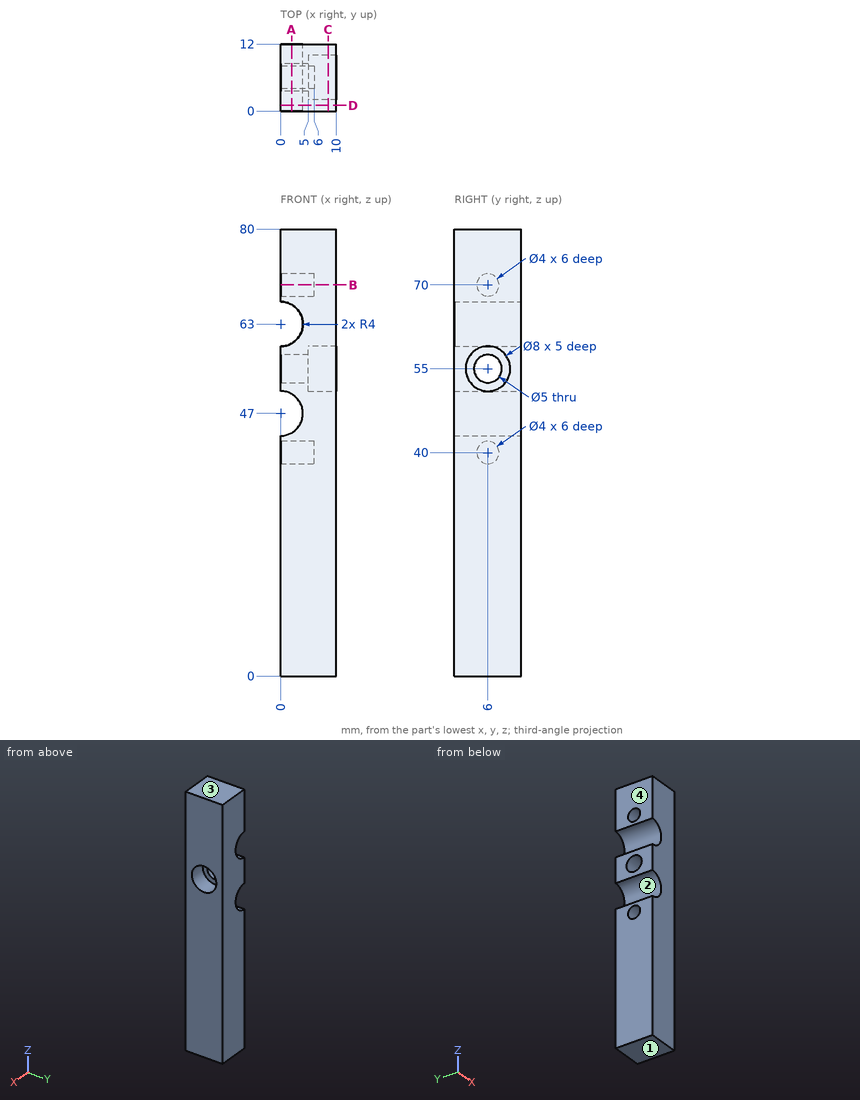
Job drawing, mm, ordinate dimensions from the low corner. One solid piece. Round coordinates to 2 decimals unless told otherwise and drop trailing zeros. Loops run counter-clockwise (first coordinate to the right, second up) from the corner with the lowest first, then second, coordinate; pieces in that order, holes last. Notation, with made-up numbers: (30.25, -18.5) -> (43.25, -18.5) arc R25 cw to (43.25, -0.5) -> close; hole circle Ø1 at (45.25, -34.5). An arc over 180 degrees is marked (long way). Use a Markdown table: item, result.
1) Cut at C-C, the plane x = 8.5. List the corners of the cut face in (y, z).
The answers:
| item | result |
|---|---|
| outline | (0, 0) -> (12, 0) -> (12, 80) -> (0, 80) -> close; hole circle Ø8 at (6, 55) |
2) Drop a flat-ended pin along its axis: pin 1 Ø6 at (y, z) = (6, 55) entering from +X. Give the stop position or say it passes through.
The answers:
| item | result |
|---|---|
| pin 1 | stops at x = 5 |
3) Cut at A-A, the plane x = 2. List the corners of the cut face in (y, z).
The answers:
| item | result |
|---|---|
| outline | (0, 0) -> (12, 0) -> (12, 43.54) -> (0, 43.54) -> close; (0, 50.46) -> (12, 50.46) -> (12, 59.54) -> (0, 59.54) -> close; (0, 66.46) -> (12, 66.46) -> (12, 80) -> (0, 80) -> close; hole circle Ø5 at (6, 55); hole circle Ø4 at (6, 40); hole circle Ø4 at (6, 70) |
4) Cut at B-B, the plane z = 70. List the corners of the cut face in (x, y).
The answers:
| item | result |
|---|---|
| outline | (0, 0) -> (10, 0) -> (10, 12) -> (0, 12) -> (0, 8) -> (6, 8) -> (6, 4) -> (0, 4) -> close |
5) Cut at D-D, the plane y = 1. List the corners of the cut face in (x, z), and give its area (3 significant figures).
The answers:
| item | result |
|---|---|
| outline | (0, 0) -> (10, 0) -> (10, 80) -> (0, 80) -> (0, 67) arc R4 cw to (0, 59) -> (0, 51) arc R4 cw to (0, 43) -> close |
| area | 750 mm2 |
6) Pull direction Z, two halves, no side cores. Call the marked faces 1, 2, 3 and 4: pulls with the +Z half, pulls with the -Z half, needs draft (parallel to the pull), parting line crosses it, or undercut.
The answers:
| item | result |
|---|---|
| face 1 | pulls with the -Z half |
| face 2 | undercut |
| face 3 | pulls with the +Z half |
| face 4 | needs draft |
7) Probe line 1 (Y direction, x = 4.75, z = 56.5); line 2 (Z direction, x = 0.5, y = 9); line 3 (Z direction, x = 3, y = 11). List the from-to ranges inside material, lowest first. Write a range as [from, to].
The answers:
| item | result |
|---|---|
| line 1 | y = [0, 4], [8, 12] |
| line 2 | z = [0, 43.03], [50.97, 59.03], [66.97, 80] |
| line 3 | z = [0, 44.35], [49.65, 60.35], [65.65, 80] |
